Design review of the part built by this model. Coordinates are the model's own, in mm. Coordinates: 2 decimals unless noted, no trailing zeros. Loops run counter-clockwise (first coordinate to the right, second up) from the corner with the lowest first, then second, coordinate; pieces in that order, holes last. Notation, with made-up numbers: (18.5, 64.25) -> (51.5, 64.25) arc R34 ccw to (51.5, 95.25) -> close; hole circle Ø9 at (79, 41.5). An arc over 180 degrees is marked (long way). Use CSV: the item, a comma, the result in double quotes.
```python
from build123d import *

# Parameters (mm, degrees)
F1_R     = 48.5
F2_DEPTH = 15
F5_R     = 12.5
F6_DEPTH = 15


with BuildPart() as f2:
    # F1 (on face) → F2 (new body)
    with BuildSketch(Plane.XY):
        Circle(F1_R)
    extrude(amount=F2_DEPTH)

    # F3 (on Front) → F4 (revolve, cut)
    with BuildSketch(Plane.XZ):
        with BuildLine():
            ThreePointArc((47.5, 7.5), (48.5, 6.5), (49.5, 7.5))
            ThreePointArc((49.5, 7.5), (48.5, 8.5), (47.5, 7.5))
        make_face()
    revolve(axis=Axis((0, 0, 8.376576), (0, 0, 1)), mode=Mode.SUBTRACT)

    # F5 (on Top) → F6 (cut)
    with BuildSketch(Plane.XY):
        Circle(F5_R)
    extrude(amount=F6_DEPTH, mode=Mode.SUBTRACT)


solid = f2.part
```
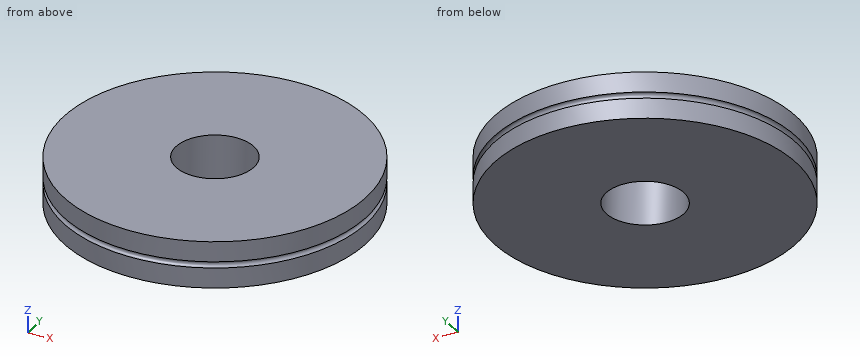
Item 1: Add section A-A (x = 0). Give the boundary of the cut face in (y, z), then the cut area to 3 significant figures.
Checked values:
outline,"(-48.5, 0) -> (-12.5, 0) -> (-12.5, 15) -> (-48.5, 15) -> (-48.5, 8.5) arc R1 cw to (-48.5, 6.5) -> close; (12.5, 0) -> (48.5, 0) -> (48.5, 6.5) arc R1 cw to (48.5, 8.5) -> (48.5, 15) -> (12.5, 15) -> close"
area,"1,080 mm^2"
Item 2: To check wall thickness, follow line 1 along Y through (x, z) = (0, 10); line 2 along X through (y, z) = (-11.5, 14); line 3 along Y through (x, z) = (-5.5, 5.25). State the ranges of each line that lie inside material, in increasing order.
Checked values:
line 1,"-48.5 to -12.5, 12.5 to 48.5"
line 2,"-47.12 to -4.9, 4.9 to 47.12"
line 3,"-48.19 to -11.22, 11.22 to 48.19"
Item 3: Clearance check with flat-ended pins moving along their axes: pin 1 (4 mm diameter, centred on y = 6, z = 12.5, fed in from -X); pin 2 (4 mm diameter, centred on x = -25.5, z = 8, fed in from -Y); pin 3 (1 mm diameter, centred on y = 12.5, z = 9.5, fed in from +X); pin 4 (12 mm diameter, centred on x = 5.5, y = 0, fed in from -Z). State where each tip first meets the part, or that it passes through.
Checked values:
pin 1,"x = -48.33"
pin 2,"y = -42.39"
pin 3,"x = 46.99"
pin 4,"through"
Item 4: Add section C-C (z = 9.75). Give the boundary of the cut face in (x, y).
Checked values:
outline,"circle Ø97 at (0, 0); hole circle Ø25 at (0, 0)"
